Build history of the part. All positions in model axes, mm. Face numbers are marked on the shaded views. Round coordinates to 2 decimals unless told otherwise and drop trailing zeros. Loops run counter-clockwise (first coordinate to the right, second up) from the corner with the lowest first, then second, coordinate; pieces in that order, holes last. Notation, with made-up numbers: M -2.75,69 L 8.25,69 A23 ccw 8.25,79 Z; hole C 61,-20 d9. An arc over 180 degrees is marked long. One line per item, written item: value.
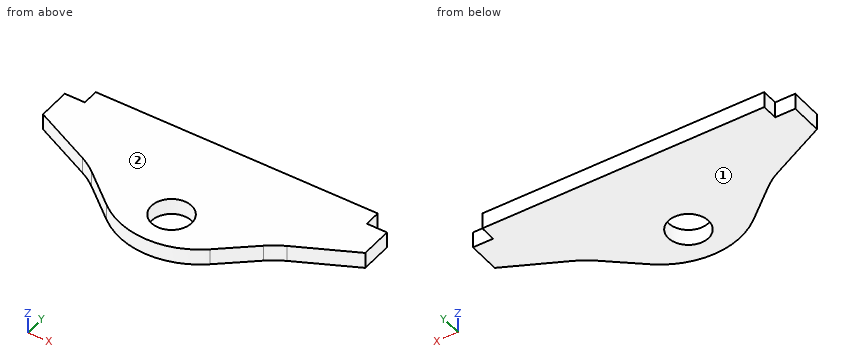
```python
from build123d import *

# Parameters (mm, degrees)
SKETCH_1_R      = 2.5
EXTRUDE_1_DEPTH = 2
FILLET_1_R      = 10


with BuildPart() as part:
    # ｽｹｯﾁ1 → ﾎﾞｽ - 押し出し1 (new body)
    with BuildSketch(Plane.XY):
        Polygon((0, -7.832443736), (11.605504985, 1.905731217), (20, 6), (20, 10), (17.5, 10), (17.5, 12), (-17.5, 12), (-17.5, 10), (-20, 10), (-20, 6), (-11.605504985, 1.905731217), align=None)
        Circle(SKETCH_1_R, mode=Mode.SUBTRACT)
    extrude(amount=EXTRUDE_1_DEPTH)

    # ﾌｨﾚｯﾄ1
    fillet_1_edges = [part.edges().sort_by_distance(p)[0] for p in [
        (11.605504985, 1.905731217, 1),
        (0, -7.832443736, 1),
        (-11.605504985, 1.905731217, 1),
    ]]
    fillet(fillet_1_edges, radius=FILLET_1_R)


solid = part.part
```
Item 1: Slice it at D-D, the plane x = 5.5. Give the cut face in (y, z), and give its area (3 significant figures).
Check values:
outline: M -3.13,0 L 12,0 L 12,2 L -3.13,2 Z
area: 30.3 mm2
Item 2: Slice it at B-B, the plane y = 0. Give the cut face in (x, z).
Check values:
outline: M -9.33,0 L -2.5,0 L -2.5,2 L -9.33,2 Z; M 2.5,0 L 9.33,0 L 9.33,2 L 2.5,2 Z
Item 3: Slice it at C-C, the plane y = 4.5. Give the cut face in (x, z), and give its area (3 significant figures).
Check values:
outline: M -16.92,0 L 16.92,0 L 16.92,2 L -16.92,2 Z
area: 67.7 mm2
Item 4: Pull direction Z, two halves, no side cores. Call the marked faces 1 and 2: pulls with the +Z half, pulls with the -Z half, needs draft (parallel to the pull), parting line crosses it, or undercut.
Check values:
face 1: pulls with the -Z half
face 2: pulls with the +Z half
Item 5: Slice it at A-A, the plane x = 0. Give the cut face in (y, z), and give its area (3 significant figures).
Check values:
outline: M -4.78,0 L -2.5,0 L -2.5,2 L -4.78,2 Z; M 2.5,0 L 12,0 L 12,2 L 2.5,2 Z
area: 23.6 mm2
Item 6: Wall check: line 1 along Y through (x, z) = (0, 0.95); line 2 along X through (y, z) = (0.5, 0.7); line 3 along X through (y, z) = (1, 0.7). Give the ranges that are in metal, low to high.
Check values:
line 1: y = -4.78 to -2.5, 2.5 to 12
line 2: x = -9.93 to -2.45, 2.45 to 9.93
line 3: x = -10.53 to -2.29, 2.29 to 10.53
